Input: dimensioned drawing with shaded views. Units: mm. Origin: part minimum x, y, z. A direction names the side the tool comes from. Round coordinates to 2 decimals unless told otherwise and drop trailing zeros. Write each loop counter-clockwise with the first axis right and the second up, starting at its lowest first coordinate (ties: lowest second). Pieces come first, ordered by that corner, then holes. Notation, with made-up numbers: M 10,54.25 L 28,54.25 A7 ccw 28,62.25 Z; hole C -19.5,-38 d5. An arc over 180 degrees is marked long. Answer in a Markdown table with one row per item. Add a question column.
Item 1: Cut plane B-B on y = 54. Return loops of the section in (x, z), and give its area (3 significant figures).
Item 2: Cut plane C-C on x = 72.5. Return loops of the section in (y, z).
Item 3: Set-up query: the marked faces 1 and 2. Return all of +Z, -Z, +X, -X, +Y, -Y with unobstructed straight access to the full face (end or side cutting, diameter ignored); none if empty.
Item 4: Cut plane A-A on z = 1. Return loops of the section in (x, y).
Item 5: Contact query for flat-ended pins moving along their axis: pin 1 (12 mm diameter, centred on x = 10.5, y = 12, fed in from +Z); pin 2 (1 mm diameter, centred on x = 90, y = 0.5, fed in from -Z). Output: stop coordinate, or through.
Item 6: Mould query, pull axis X, two halves, no side actions, for the marked faces 3, 4, 5 and 6. Classes: released by +X, released by -X, zero draft, split by the parting line, or undercut.
Item 7: Material intervals for probe 1 along X at (y, z) = (40, 10); probe 2 along Y at (x, z) = (11.5, 10.75); probe 3 along X at (y, z) = (40.5, 1.75), sorted ascending.
Item 8: Cut plane D-D on z = 6.5. Return loops of the section in (x, y), and give its area (3 significant figures).
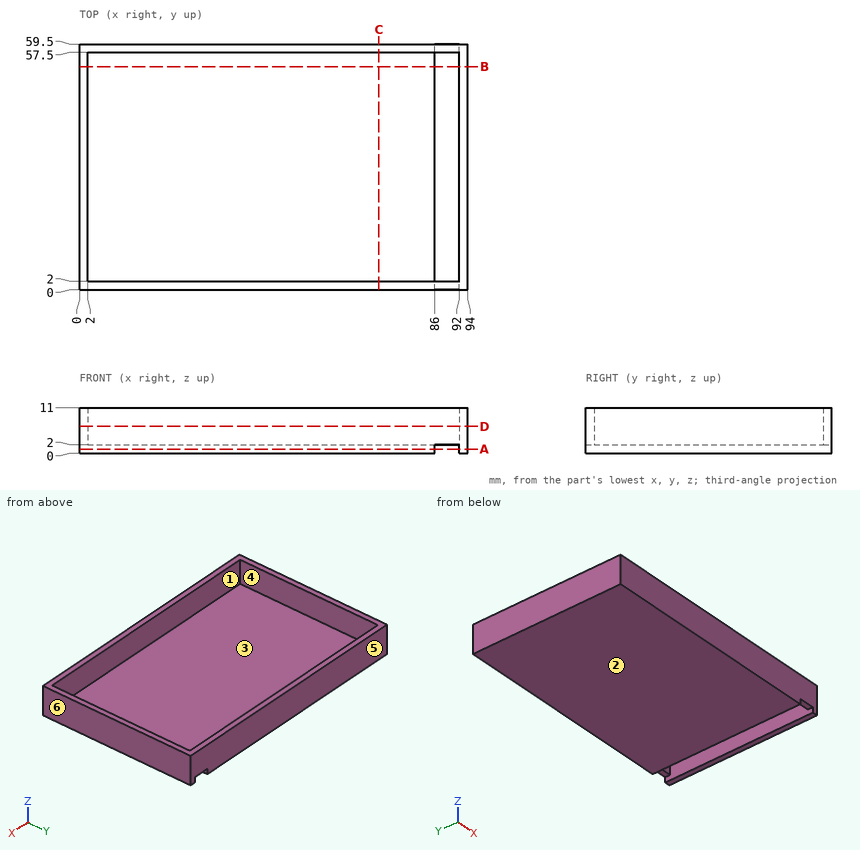
Results below:
| question | item | result |
|---|---|---|
| 1 | outline | M 0,0 L 86,0 L 86,2 L 2,2 L 2,11 L 0,11 Z; M 92,0 L 94,0 L 94,11 L 92,11 Z |
| 1 | area | 212 mm2 |
| 2 | outline | M 0,0 L 59.5,0 L 59.5,11 L 57.5,11 L 57.5,2 L 2,2 L 2,11 L 0,11 Z |
| 3 | face 1 | +Z |
| 3 | face 2 | -Z, +X, -X, +Y, -Y |
| 4 | outline | M 0,0 L 86,0 L 86,59.5 L 0,59.5 Z; M 92,0 L 94,0 L 94,59.5 L 92,59.5 Z |
| 5 | pin 1 | z = 2 |
| 5 | pin 2 | z = 2 |
| 6 | face 3 | undercut |
| 6 | face 4 | undercut |
| 6 | face 5 | zero draft |
| 6 | face 6 | released by +X |
| 7 | probe 1 | 0 to 2, 92 to 94 |
| 7 | probe 2 | 0 to 2, 57.5 to 59.5 |
| 7 | probe 3 | 0 to 86, 92 to 94 |
| 8 | outline | M 0,0 L 94,0 L 94,59.5 L 0,59.5 Z; hole M 2,2 L 92,2 L 92,57.5 L 2,57.5 Z |
| 8 | area | 598 mm2 |
